Source: CAD feature listing. Evaluate the final solid. Frame: model axes, mm. Face numbers are marked on the shaded views. A direction names the side the tool comes from. Give positions to 0.01 mm unless a question says otherwise; leave off trailing zeros. Write each loop counter-clockwise with the first axis right and the second up, starting at its lowest first coordinate (ties: lowest second). Pieces come first, ordered by that corner, then holes.
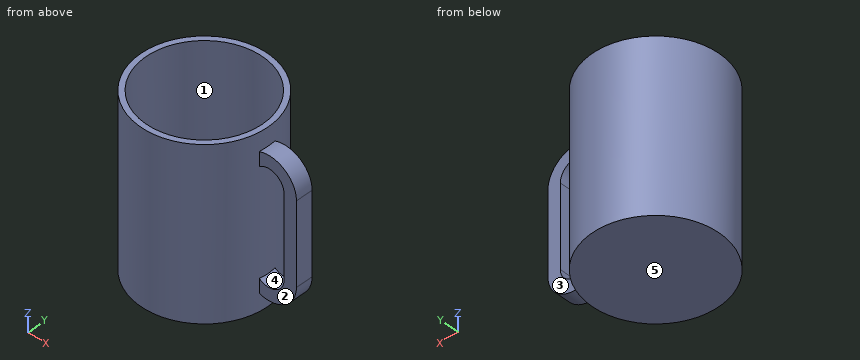
```python
from build123d import *

# Parameters (mm, degrees)
F0_R          = 38.1
F1_DEPTH      = 50.8
F1_DEPTH_BACK = 50.8
F2_R          = 34.925
F3_DEPTH      = 99.06
F5_DEPTH      = 5.08
F5_DEPTH_BACK = 5.08
F6_R          = 12.7


with BuildPart() as f1:
    # F0 (on Top) → F1 (new body, two sides)
    with BuildSketch(Plane.XY) as f1_sk:
        Circle(F0_R)
    extrude(amount=F1_DEPTH)
    extrude(f1_sk.sketch, amount=-F1_DEPTH_BACK)

    # F2 (on face) → F3 (cut)
    with BuildSketch(Plane.XY.offset(50.8)):
        Circle(F2_R)
    extrude(amount=-F3_DEPTH, mode=Mode.SUBTRACT)

    # F4 (on Front) → F5 (join, two sides)
    with BuildSketch(Plane.XZ) as f5_sk:
        with BuildLine():
            Line((60.119201, -24.80282), (60.119201, 24.239462))
            ThreePointArc((60.119201, 24.239462), (52.108585, 38.460985), (35.794442, 38.981002))
            Line((35.794442, 38.981002), (35.794442, 29.205198))
            ThreePointArc((35.794442, 29.205198), (46.078305, 33.024621), (52.648449, 24.239462))
            Line((52.648449, 24.239462), (52.648449, -24.80282))
            ThreePointArc((52.648449, -24.80282), (46.078305, -33.58798), (35.794442, -29.768556))
            Line((35.794442, -29.768556), (35.794442, -39.54436))
            ThreePointArc((35.794442, -39.54436), (52.108585, -39.024344), (60.119201, -24.80282))
        make_face()
    extrude(amount=F5_DEPTH)
    extrude(f5_sk.sketch, amount=-F5_DEPTH_BACK)

    # F6
    f6_edges = [f1.edges().sort_by_distance(p)[0] for p in [
        (-34.925, 0, -48.26),
    ]]
    fillet(f6_edges, radius=F6_R)


solid = f1.part
```
1. Cut plane D-D, the plane x = 0. Return the cut outline in (y, z) (3 decimals).
2. Cut plane C-C, the plane y = 0. Return the cut outline in (x, z) (3 decimals), then the cut area to 3 significant figures.
3. Access query for the marked faces 1 and 2. Directions: +Z, -Z, +X, -X, +Y, -Y. A direction counts if a zero-diameter tool reaches every point of the face in a straight line with its end or side. Return the directions, or none.
4. Cut plane A-A, the plane z = -5.5. Return the cut outline in (x, y) (3 decimals), then the cut area to 3 significant figures.
5. Line query: L1, parallel to Y at x = 0, z = -13.5 (3 decimals); L2, parallel to X at y = 4, z = -16; L3, parallel to Z at x = 17, y = 8.5. Output: solid intervals per line, ascending.
6. Mould query, pull axis Z, two halves, no side actions, for the marked faces 3, 4 and 5. Classes: +Z half, -Z half, draft (parallel to the pull), parting line (faces both ways), or undercut.
7. Cut plane B-B, the plane x = 44. Return the cut outline in (y, z), then the cut area to 3 significant figures.
8. Contact query for flat-ended pins moving along their axis: P1, Ø6.5, axis at x = 51.5, z = 4.5, coming from the -Y side; P2, Ø10, axis at x = -10.5, z = 23.5, coming from the -Y side; P3, Ø24.5, axis at x = 43.5, z = 12, coming from the +Y side. Output: stop coordinate, or through.
Response values:
1. outline: (-38.1, -50.8) - (38.1, -50.8) - (38.1, 50.8) - (34.925, 50.8) - (34.925, -35.56) arc R12.7 cw to (22.225, -48.26) - (-22.225, -48.26) arc R12.7 cw to (-34.925, -35.56) - (-34.925, 50.8) - (-38.1, 50.8) - close
2. outline: (-38.1, -50.8) - (38.1, -50.8) - (38.1, -40.534) arc R16.629 ccw to (60.119, -24.803) - (60.119, 24.239) arc R16.629 ccw to (38.1, 39.971) - (38.1, 50.8) - (34.925, 50.8) - (34.925, -35.56) arc R12.7 cw to (22.225, -48.26) - (-22.225, -48.26) arc R12.7 cw to (-34.925, -35.56) - (-34.925, 50.8) - (-38.1, 50.8) - close; hole (38.1, -32.207) arc R9.159 ccw to (52.648, -24.803) - (52.648, 24.239) arc R9.159 ccw to (38.1, 31.644) - close
2. area: 1,640 mm2
3. face 1: +Z
3. face 2: +Z, -Z, +X, -Y
4. outline: circle Ø76.2 at (0, 0); (52.648, -5.08) - (60.119, -5.08) - (60.119, 5.08) - (52.648, 5.08) - close; hole circle Ø69.85 at (0, 0)
4. area: 804 mm2
5. L1: y = -38.1 to -34.925, 34.925 to 38.1
5. L2: x = -37.89 to -34.7, 34.7 to 37.89, 52.65 to 60.12
5. L3: z = -50.8 to -48.26
6. face 3: draft
6. face 4: undercut
6. face 5: -Z half
7. outline: (-5.08, -41.42) - (5.08, -41.42) - (5.08, -33.95) - (-5.08, -33.95) - close; (-5.08, 33.38) - (5.08, 33.38) - (5.08, 40.86) - (-5.08, 40.86) - close
7. area: 152 mm2
8. P1: stops at y = -5.08
8. P2: stops at y = -37.7
8. P3: stops at y = 21.8
